The listing builds one solid part. Answer for the finished solid, in the listing's coordinates (mm). A direction names the side the tool comes from. Round coordinates to 2 decimals unless told otherwise and drop trailing zeros. Loops run counter-clockwise (first coordinate to the right, second up) from the corner with the lowest first, then second, coordinate; pieces in that order, holes last. Notation, with made-up numbers: (-8.75, -12.75) -> (2.25, -12.75) arc R19 cw to (2.25, 9.25) -> close; hole circle Ø3 at (84, 43). An arc over 180 degrees is marked (long way). Answer in a Markdown table with one row per item. Add a question column.
Autodesk Inventor part; units mm, degrees
ref_plane "YZ Plane" through (0, 0, 0) normal (1, 0, 0) x (0, 1, 0)
ref_plane "XZ Plane" through (0, 0, 0) normal (0, 1, 0) x (-1, 0, 0)
ref_plane "XY Plane" through (0, 0, 0) normal (0, 0, 1) x (1, 0, 0)
sketch "Sketch1" plane through (0, 0, 0) normal (0, 0, 1) x (1, 0, 0)
  line L0 (-125, 9.5) -> (125, 9.5)
  circle A0 centre (125, 0) radius 9.5 construction
  arc A1 (125, -9.5) -> (125, 9.5) centre (125, 0) ccw
  line L1 (-125, -9.5) -> (125, -9.5)
  arc A2 (-125, 9.5) -> (-125, -9.5) centre (-125, 0) ccw
  line L2 (125, 8.5) -> (-125, 8.5)
  arc A3 (-125, 8.5) -> (-125, -8.5) centre (-125, 0) ccw
  line L3 (-125, -8.5) -> (125, -8.5)
  arc A4 (125, -8.5) -> (125, 8.5) centre (125, 0) ccw
  point P0 (0, 0)
  point P1 (0, 9.5)
  dimension "d0" = 250
  dimension "d3" = 1
  dimension "d8" = 8.5
  dimension "d9" = 17
extrude "Extrusion1" add sketch "Sketch1" along normal mid plane 48
properties part number "Conveyor_003_001" material "Rubber"
Item 1: A flat-ended cylindrical pin translates along its axis: P1, Ø4, axis at x = -45.5, y = -6, coming from the +Z side. Find the tip coordinate at first contact, or state that the pin passes through.
Item 2: Section A-A, the plane z = -9 is taken. Write down the section's boundary in (x, y).
Item 3: For faces 4 (the flat face through (2, 8.5, 0)), 5 (the flat face through (-2, -9.5, 0)), determine the directions among +Z, -Z, +X, -X, +Y, -Y from which every point of the face is accessible in a straight line to the end or side of a thin tool.
Item 4: Section B-B, the plane y = 0 is taken. Write down the section's boundary in (x, z).
Item 5: Section C-C, the plane x = -83 is taken. Write down the section's boundary in (y, z).
Item 6: Consider L1, parallel to Y at x = -48, z = 22.5; L2, parallel to X at y = 0.75, z = 3; L3, parallel to X at y = 7.75, z = 10. Determine where each line is inside the solid, lowest interval first. Write a range as from..to.
Item 7: The mould has two halves that part along Y. Classify faces 1 (the flat face through (-2, 9.5, 0)), 2 (the flat face through (-1, 9, 24)), 3 (the cylindrical face through (133.498, 0.187, -0.336)): +Y half, -Y half, draft (parallel to the pull), parting line (faces both ways), or undercut.
Here are the results:
| question | item | result |
|---|---|---|
| 1 | P1 | passes through |
| 2 | outline | (-125, -9.5) -> (125, -9.5) arc R9.5 ccw to (125, 9.5) -> (-125, 9.5) arc R9.5 ccw to start; hole (-125, -8.5) -> (125, -8.5) arc R8.5 ccw to (125, 8.5) -> (-125, 8.5) arc R8.5 ccw to start |
| 3 | face 4 | +Z, -Z |
| 3 | face 5 | +Z, -Z, +X, -X, -Y |
| 4 | outline | (-134.5, -24) -> (-133.5, -24) -> (-133.5, 24) -> (-134.5, 24) -> close; (133.5, -24) -> (134.5, -24) -> (134.5, 24) -> (133.5, 24) -> close |
| 5 | outline | (-9.5, -24) -> (-8.5, -24) -> (-8.5, 24) -> (-9.5, 24) -> close; (8.5, -24) -> (9.5, -24) -> (9.5, 24) -> (8.5, 24) -> close |
| 6 | L1 | y = -9.5..-8.5, 8.5..9.5 |
| 6 | L2 | x = -134.47..-133.47, 133.47..134.47 |
| 6 | L3 | x = -130.49..-128.49, 128.49..130.49 |
| 7 | face 1 | +Y half |
| 7 | face 2 | draft |
| 7 | face 3 | undercut |
